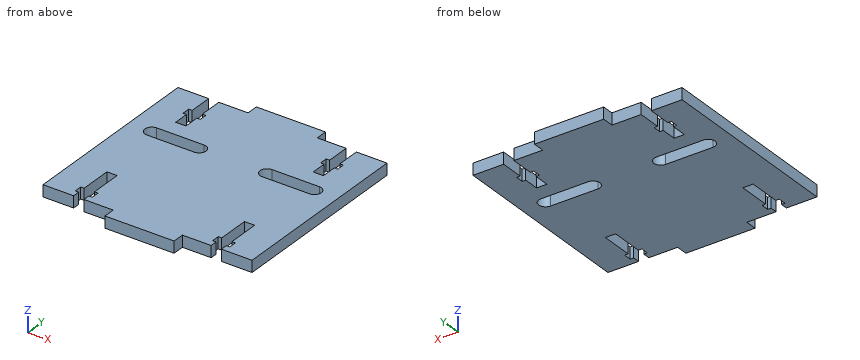
from build123d import *

# Parameters (mm, degrees)
SKETCH1_W           = 90
SKETCH1_H           = 82
BOSS_EXTRUDE1_DEPTH = 5
SKETCH4_W           = 29.8
SKETCH4_H           = 5
BOSS_EXTRUDE2_DEPTH = 5
CUT_EXTRUDE1_DEPTH  = 10
CUT_EXTRUDE2_DEPTH  = 10


with BuildPart() as part:
    # Sketch1 → Boss-Extrude1 (new body)
    with BuildSketch(Plane.XY):
        Rectangle(SKETCH1_W, SKETCH1_H)
    extrude(amount=BOSS_EXTRUDE1_DEPTH)

    # Sketch4 → Boss-Extrude2 (add)
    with BuildSketch(Plane.XY.offset(5)):
        with Locations((0.1, 43.5)):
            Rectangle(SKETCH4_W, SKETCH4_H)
    boss_extrude2 = extrude(amount=-BOSS_EXTRUDE2_DEPTH)

    # Mirror1: Boss-Extrude2 across plane
    add(boss_extrude2.mirror(Plane(origin=(0, 0, 0), x_dir=(0, 0, 1), z_dir=(0, -1, 0))))

    # Sketch5 → Cut-Extrude1 (cut)
    with BuildSketch(Plane.XY.offset(5)):
        Polygon((27.39999999, 41), (27.39999999, 31), (25.89999999, 31), (25.89999999, 27.6), (27.39999999, 27.6), (27.39999999, 21), (31.79999999, 21), (31.79999999, 27.6), (33.29999999, 27.6), (33.29999999, 31), (31.79999999, 31), (31.79999999, 41), align=None)
        Polygon((-27.39999999, 27.6), (-27.39999999, 21), (-31.79999999, 21), (-31.79999999, 27.6), (-33.29999999, 27.6), (-33.29999999, 31), (-31.79999999, 31), (-31.79999999, 41), (-27.39999999, 41), (-27.39999999, 31), (-25.89999999, 31), (-25.89999999, 27.6), align=None)
        Polygon((-27.4, -38), (-27.4, -41), (-31.8, -41), (-31.8, -38), (-33.3, -38), (-33.3, -34.6), (-31.8, -34.6), (-31.8, -20.8), (-27.4, -20.8), (-27.4, -34.6), (-25.9, -34.6), (-25.9, -38), align=None)
        Polygon((31.8, -41), (31.8, -38), (33.3, -38), (33.3, -34.6), (31.8, -34.6), (31.8, -20.8), (27.4, -20.8), (27.4, -34.6), (25.9, -34.6), (25.9, -38), (27.4, -38), (27.4, -41), align=None)
    extrude(amount=-CUT_EXTRUDE1_DEPTH, mode=Mode.SUBTRACT)

    # Sketch6 → Cut-Extrude2 (cut)
    with BuildSketch(Plane.XY.offset(5)):
        with BuildLine():
            Line((-14.6, 14), (-35, 14))
            ThreePointArc((-35, 14), (-38, 11), (-35, 8))
            Line((-35, 8), (-14.6, 8))
            ThreePointArc((-14.6, 8), (-11.6, 11), (-14.6, 14))
        make_face()
        with BuildLine():
            Line((35, 8), (14.6, 8))
            ThreePointArc((14.6, 8), (11.6, 11), (14.6, 14))
            Line((14.6, 14), (35, 14))
            ThreePointArc((35, 14), (38, 11), (35, 8))
        make_face()
    extrude(amount=-CUT_EXTRUDE2_DEPTH, mode=Mode.SUBTRACT)


solid = part.part
Work out the finished part from the listing and answer in its coordinate system (mm). Give positions to 0.01 mm unless a question says otherwise; leave off trailing zeros. Write each loop counter-clockwise with the first axis right and the second up, starting at its lowest first coordinate (ties: lowest second). Pieces come first, ordered by that corner, then holes.
Q1. Straight lines are drawn through the part: L1, parallel to X at y = -36.5, z = 2.95; L2, parallel to X at y = 35, z = 1.4; L3, parallel to Y at x = -22, z = 3.2. For each, find the intervals that lie inside material, in ascending order.
Answer:
L1: x = -45 to -33.3, -25.9 to 25.9, 33.3 to 45
L2: x = -45 to -31.8, -27.4 to 27.4, 31.8 to 45
L3: y = -41 to 8, 14 to 41
Q2. The part is cut by section D-D on y = 11. Give the vertices of the cut face in (x, z).
Answer:
outline: (-45, 0) - (-38, 0) - (-38, 5) - (-45, 5) - close; (-11.6, 0) - (11.6, 0) - (11.6, 5) - (-11.6, 5) - close; (38, 0) - (45, 0) - (45, 5) - (38, 5) - close
Q3. Given pin 1 (1.5 mm diameter, centred on x = 19, z = 3.5, fed in from -Y); pin 2 (1.5 mm diameter, centred on x = -23.5, z = 2, fed in from +Y), each flat-ended and moving along its own axis, determine where each tip first touches the part or whether it passes through.
Answer:
pin 1: stops at y = -41
pin 2: stops at y = 41
Q4. The part is cut by section C-C on z = 3.8. State how many separate pieces and enclosed holes the cut face has, and give its area (3 significant figures).
Answer:
separate pieces: 1
enclosed holes: 2
area: 6,980 mm2
Q5. The part is cut by section B-B on y = -28. Give the vertices of the cut face in (x, z), and give its area (3 significant figures).
Answer:
outline: (-45, 0) - (-31.8, 0) - (-31.8, 5) - (-45, 5) - close; (-27.4, 0) - (27.4, 0) - (27.4, 5) - (-27.4, 5) - close; (31.8, 0) - (45, 0) - (45, 5) - (31.8, 5) - close
area: 406 mm2
Q6. The part is cut by section A-A on x = 17. Give the vertices of the cut face in (y, z).
Answer:
outline: (-41, 0) - (8, 0) - (8, 5) - (-41, 5) - close; (14, 0) - (41, 0) - (41, 5) - (14, 5) - close
